Check sheet for the modelled part. Datum: model origin and axes. Units: mm. A direction names the side the tool comes from. Round coordinates to 2 decimals unless told otherwise and drop trailing zeros. Write each loop counter-clockwise with the first axis right and the second up, starting at its lowest first coordinate (ties: lowest second). Pieces come first, ordered by that corner, then holes.
Item 1: Depth check by flat-ended pin: pin 1 (8 mm diameter, centred on x = -207, z = -121.5, fed in from +Y); pin 2 (2 mm diameter, centred on x = 3.5, y = 20.5, fed in from +Z); pin 3 (2 mm diameter, centred on x = -149, y = 2, fed in from +Z). Enter the tip coordinate at first touch or a pass-through.
Item 2: Material ranges on line 1 along X through (y, z) = (-4.5, 0); line 2 along Z through (x, y) = (0, -2.5); line 3 along Y through (x, z) = (-226, 270), recorded low to high.
Item 3: Set-up check for faces 5 (the cylindrical face through (335.73, 12.88, -257.06)), 6 (the flat face through (381, 10, 72)): record each of +Z, -Z, +X, -X, +Y, -Y from which the full face is reachable in a straight line by a thin tool's end or side.
Item 4: Section check A-A, the plane z = 0. Record the cut outline in (x, y).
Item 5: Release check for a two-part mould opening along Y. For faces 1 (the flat face through (5, -6.35, 72)), 2 (the cylindrical face through (-75.152, 12.979, -285.753)), 3 (the cylindrical face through (12.4, -3.22, -2.75)), 4 (the cylindrical face through (361.953, 12.979, 82.531)) record: pulls with the +Y half, pulls with the -Y half, needs draft (parallel to the pull), parting line crosses it, or undercut.
Item 6: Section check D-D, the plane x = -177. Record the cut outline in (y, z).
Item 7: Section check C-C, the plane y = 12.7. Record the cut outline in (x, z).
Item 8: Section check B-B, the plane x = 0. Record the cut outline in (y, z), plus the area to 3 significant figures.
Autodesk Inventor part; units mm, degrees
ref_plane "Work Plane3" through (-381, 0, 304.8) normal (0, 0, 1) x (1, 0, 0)
ref_plane "Work Plane4" through (0, 12.7, 0) normal (0, 1, 0) x (1, 0, 0)
ref_plane "YZ Plane" through (0, 0, 0) normal (1, 0, 0) x (0, 1, 0)
sketch "Sketch1" plane through (0, 0, 0) normal (0, 1, 0) x (-1, 0, 0)
  line L0 (-381, 304.8) -> (-381, -304.8)
  line L1 (-381, -304.8) -> (381, -304.8)
  line L2 (381, -304.8) -> (381, 304.8)
  line L3 (381, 304.8) -> (-381, 304.8)
  line L4 (-381, 304.8) -> (381, -304.8) construction
  line L5 (-381, -304.8) -> (381, 304.8) construction
  point P0 (0, 0)
  dimension "width" = 609.6
  dimension "length" = 762
extrude "Extrusion1" add sketch "Sketch1" against normal blind 6.35
ref_plane "Work Plane3" through (-381, 0, 304.8) normal (0, 0, 1) x (1, 0, 0)
sketch "Sketch5" plane through (-381, 0, 304.8) normal (0, 0, 1) x (1, 0, 0)
  line L0 (762, 0) -> (755.65, 0)
  line L1 (755.65, 25.4) -> (762, 25.4)
  line L2 (762, 25.4) -> (762, 0)
  arc A0 (755.65, 25.4) -> (755.65, 0) centre (755.65, 12.7) ccw
  point P0 (381, 0)
  dimension "d16" = 25.4
ref_plane "Work Plane4" through (0, 12.7, 0) normal (0, 1, 0) x (1, 0, 0)
sketch "Sketch6" plane through (0, 12.7, 0) normal (0, 1, 0) x (1, 0, 0)
  line L0 (-381, 304.8) -> (381, 304.8) construction
  line L1 (222.25, 304.8) -> (222.25, 146.05) construction
  line L2 (222.25, 146.05) -> (381, 146.05) construction
  line L3 (381, 304.8) -> (381, -304.8) construction
  arc A0 (368.3, 146.05) -> (222.25, 292.1) centre (222.25, 146.05) ccw
  line L4 (222.25, 292.1) -> (-381, 292.1)
  line L5 (-381, -304.8) -> (-381, 304.8)
  line L6 (368.3, 146.05) -> (368.3, -304.8)
  line L7 (381, -304.8) -> (-381, -304.8)
  point P0 (0, 0)
  dimension "d20" = 158.75
  dimension "diameterOfFrisbee" = 292.1
sweep "Sweep2" add profiles "Sketch5" path "Sketch6" path curves L6 A0 L4
sketch "Sketch7" plane through (0, 0, 0) normal (0, 1, 0) x (1, 0, 0)
  point P0 (0, 0)
  point P1 (0, 0)
hole "Hole1" at (0, 0, 0) direction (0, -1, 0) diameter 25.4 end through all
properties part number "ShooterBase" material "Wood (Birch)"
Values found:
1. pin 1: stops at y = 0
1. pin 2: stops at z = -287.72
1. pin 3: stops at z = -290.25
2. line 1: x = -381 to -12.7, 12.7 to 381
2. line 2: z = -304.8 to -12.7, 12.7 to 304.8
2. line 3: y = -6.35 to 0
3. face 5: -Z, +X, +Y
3. face 6: +Z, -Z, +X, +Y, -Y
4. outline: (-381, -6.35) - (-12.7, -6.35) - (-12.7, 0) - (-381, 0) - close; (12.7, -6.35) - (381, -6.35) - (381, 25.4) - (374.65, 25.4) arc R12.7 ccw to (374.65, 0) - (12.7, 0) - close
5. face 1: pulls with the -Y half
5. face 2: undercut
5. face 3: needs draft
5. face 4: undercut
6. outline: (-6.35, -304.8) - (25.4, -304.8) - (25.4, -298.45) arc R12.7 ccw to (0, -298.45) - (0, 304.8) - (-6.35, 304.8) - close
7. outline: (-381, -304.8) - (222.25, -304.8) arc R158.75 ccw to (381, -146.05) - (381, 304.8) - (361.95, 304.8) - (361.95, -146.05) arc R139.7 cw to (222.25, -285.75) - (-381, -285.75) - close
8. outline: (-6.35, -304.8) - (25.4, -304.8) - (25.4, -298.45) arc R12.7 ccw to (0, -298.45) - (0, -12.7) - (-6.35, -12.7) - close; (-6.35, 12.7) - (0, 12.7) - (0, 304.8) - (-6.35, 304.8) - close
8. area: 4,120 mm2
